Drawing for the job (mm, zero at the part's lowest x, y, z). Give positions to 0.01 mm unless a question says otherwise; leave off trailing zeros. Write each loop counter-clockwise with the first axis right and the second up, starting at its lowest first coordinate (ties: lowest second). Pieces come first, ordered by that corner, then holes. Notation, with made-up numbers: (28, 60) - (48, 60) arc R23 ccw to (48, 81) - close; hole circle Ø3 at (-34, 65.5). An arc over 180 degrees is marked (long way). Answer as a JSON object with one key per item and string values. Group by question number.
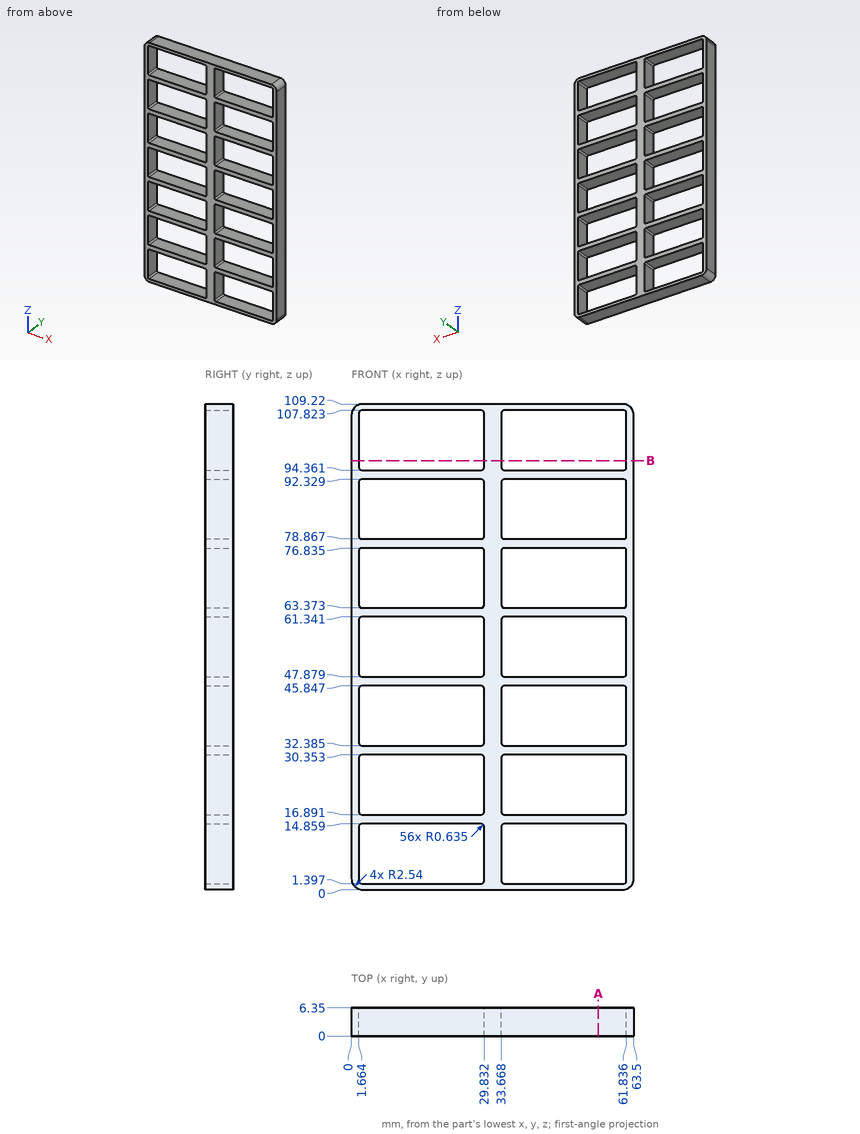
1) Probe line 1 (X direction, y = 3.75, z = 71.5); line 2 (X direction, y = 2.75, z = 94.5) (1 decimal). List the from-to ranges inside material, lowest first.
2) Band-saw the part on A-A (x = 55.5). State how many separate pieces and enclosed holes the cut face has.
3) Band-saw the part on B-B (z = 96.5). List the corners of the cut face in (x, y), plus the area to 3 significant figures.
Verdict:
{
 "1": {"line 1": "0 to 1.66, 29.83 to 33.67, 61.84 to 63.5", "line 2": "0 to 1.9, 29.6 to 33.9, 61.6 to 63.5"},
 "2": {"separate pieces": "8", "enclosed holes": "0"},
 "3": {"outline": "(0, 0) - (1.66, 0) - (1.66, 6.35) - (0, 6.35) - close; (29.83, 0) - (33.67, 0) - (33.67, 6.35) - (29.83, 6.35) - close; (61.84, 0) - (63.5, 0) - (63.5, 6.35) - (61.84, 6.35) - close", "area": "45.5 mm2"}
}
